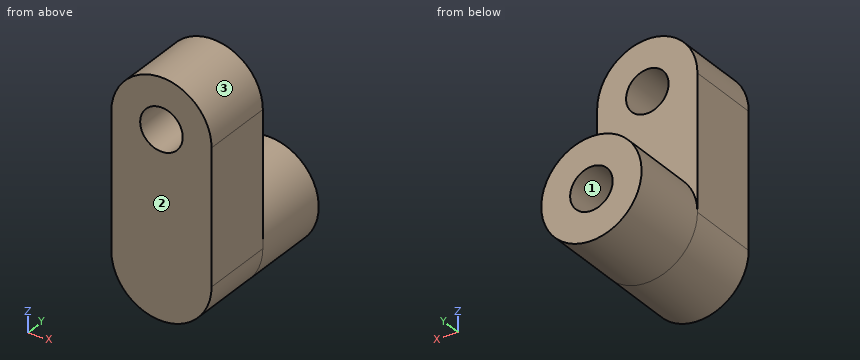
```python
from build123d import *

# Parameters (mm, degrees)
BOSS_EXTRUDE1_DEPTH             = 5.5
SKETCH2_R                       = 1.59
CUT_EXTRUDE1_DEPTH              = 13.013013777
SKETCH3_R                       = 3.75
BOSS_EXTRUDE2_DEPTH             = 6
BOSS_EXTRUDE2_DIRECTION_2_REACH = 14.013
SKETCH4_R                       = 1.59
CUT_EXTRUDE2_DEPTH              = 10


with BuildPart() as part:
    # Sketch1 → Boss-Extrude1 (new body)
    with BuildSketch(Plane(origin=(0, 0, 0), x_dir=(1, 0, 0), z_dir=(0, 1, 0))):
        with BuildLine():
            Line((-3.75, 10), (-3.75, 0))
            ThreePointArc((-3.75, 0), (0, -3.75), (3.75, 0))
            Line((3.75, 0), (3.75, 10))
            Line((3.75, 10), (-3.75, 10))
        make_face()
    extrude(amount=BOSS_EXTRUDE1_DEPTH)

    # Sketch2 → Cut-Extrude1 (cut, through all)
    with BuildSketch(Plane(origin=(0, 5.5, 0), x_dir=(1, 0, 0), z_dir=(0, 1, 0))):
        with Locations(Location((0, 0, 0), (0, 0, 270))):
            Circle(SKETCH2_R)
    extrude(amount=-CUT_EXTRUDE1_DEPTH, mode=Mode.SUBTRACT)

    # Sketch3 → Boss-Extrude2 (add)
    with BuildSketch(Plane(origin=(0, 5.5, 0), x_dir=(1, 0, 0), z_dir=(0, 1, 0))):
        with Locations(Location((0, 10, 0), (0, 0, 270))):
            Circle(SKETCH3_R)
    extrude(amount=BOSS_EXTRUDE2_DEPTH)

    # Boss-Extrude2 direction 2: up to this face of the body (flat: up to its plane)
    boss_extrude2_direction_2_end = Plane(part.part.faces().sort_by_distance((0, 0, -3.812169899))[0])
    # Sketch3 → Boss-Extrude2 direction 2 (add, up to the picked face)
    with BuildSketch(Plane(origin=(0, 5.5, 0), x_dir=(1, 0, 0), z_dir=(0, 1, 0)), mode=Mode.PRIVATE) as boss_extrude2_direction_2_sk1:
        with Locations(Location((0, 10, 0), (0, 0, 270))):
            Circle(SKETCH3_R)
    boss_extrude2_direction_2_tool1 = split(extrude(boss_extrude2_direction_2_sk1.sketch, amount=-BOSS_EXTRUDE2_DIRECTION_2_REACH, mode=Mode.PRIVATE), bisect_by=boss_extrude2_direction_2_end, keep=Keep.BOTH, mode=Mode.PRIVATE)
    add(boss_extrude2_direction_2_tool1.solids().sort_by(Axis((0, 5.5, -10), (0, -1, 0)))[0])

    # Sketch4 → Cut-Extrude2 (cut)
    with BuildSketch(Plane(origin=(0, 11.5, 0), x_dir=(1, 0, 0), z_dir=(0, 1, 0))):
        with Locations(Location((0, 10, 0), (0, 0, 270))):
            Circle(SKETCH4_R)
    extrude(amount=-CUT_EXTRUDE2_DEPTH, mode=Mode.SUBTRACT)


solid = part.part
```
Design review of the part built by this model. Coordinates are the model's own, in mm. Face numbers are marked on the shaded views. Coordinates: 2 decimals unless noted, no trailing zeros. Loops run counter-clockwise (first coordinate to the right, second up) from the corner with the lowest first, then second, coordinate; pieces in that order, holes last. Notation, with made-up numbers: (-10, 71.5) - (19, 71.5) arc R19 cw to (19, 102.5) - close; hole circle Ø8 at (-26, -8.5). An arc over 180 degrees is marked (long way). Use CSV: the item, a comma, the result in double quotes. Start each with the question number.
1) Consider section C-C on y = 6.25. Write out the cut boundary in (x, z), then the cut area to 3 significant figures.
2) Wall thickness on L1, parallel to X at y = 9.5, z = -10; L2, parallel to Z at x = -0.75, y = 1.75: over which ranges is each line inside the solid? List them lowest first. Write a range as from..to.
3) For pin 1 Ø2 at (x, z) = (-0.5, -5) entering from +Y, flat-tipped, find the tip position at first contact; note if it passes through.
4) Consider section A-A on x = 0. Write out the cut boundary in (y, z), then the cut area to 3 significant figures.
5) Consider section D-D on z = -7. Write out the cut boundary in (x, y).
6) The part is to be moulded in two halves that separate along Z. For the marked faces 1, 2 and 3, say which applies: +Z half, -Z half, draft (parallel to the pull), parting line (faces both ways), or undercut.
7) Consider section B-B on z = 1. Write out the cut boundary in (x, y).
Geometry says:
1,outline,"circle Ø7.5 at (0, -10); hole circle Ø3.18 at (0, -10)"
1,area,"36.2 mm^2"
2,L1,"-3.75..-1.59, 1.59..3.75"
2,L2,"-13.67..-11.4, -8.6..-1.4, 1.4..3.67"
3,pin 1,"y = 5.5"
4,outline,"(0, -13.75) - (11.5, -13.75) - (11.5, -11.59) - (1.5, -11.59) - (1.5, -8.41) - (11.5, -8.41) - (11.5, -6.25) - (5.5, -6.25) - (5.5, -1.59) - (0, -1.59) - close; (0, 1.59) - (5.5, 1.59) - (5.5, 3.75) - (0, 3.75) - close"
4,area,"92.0 mm^2"
5,outline,"(-3.75, 0) - (3.75, 0) - (3.75, 5.5) - (2.25, 5.5) - (2.25, 11.5) - (-2.25, 11.5) - (-2.25, 5.5) - (-3.75, 5.5) - close"
6,face 1,"undercut"
6,face 2,"draft"
6,face 3,"+Z half"
7,outline,"(-3.61, 0) - (-1.24, 0) - (-1.24, 5.5) - (-3.61, 5.5) - close; (1.24, 0) - (3.61, 0) - (3.61, 5.5) - (1.24, 5.5) - close"
